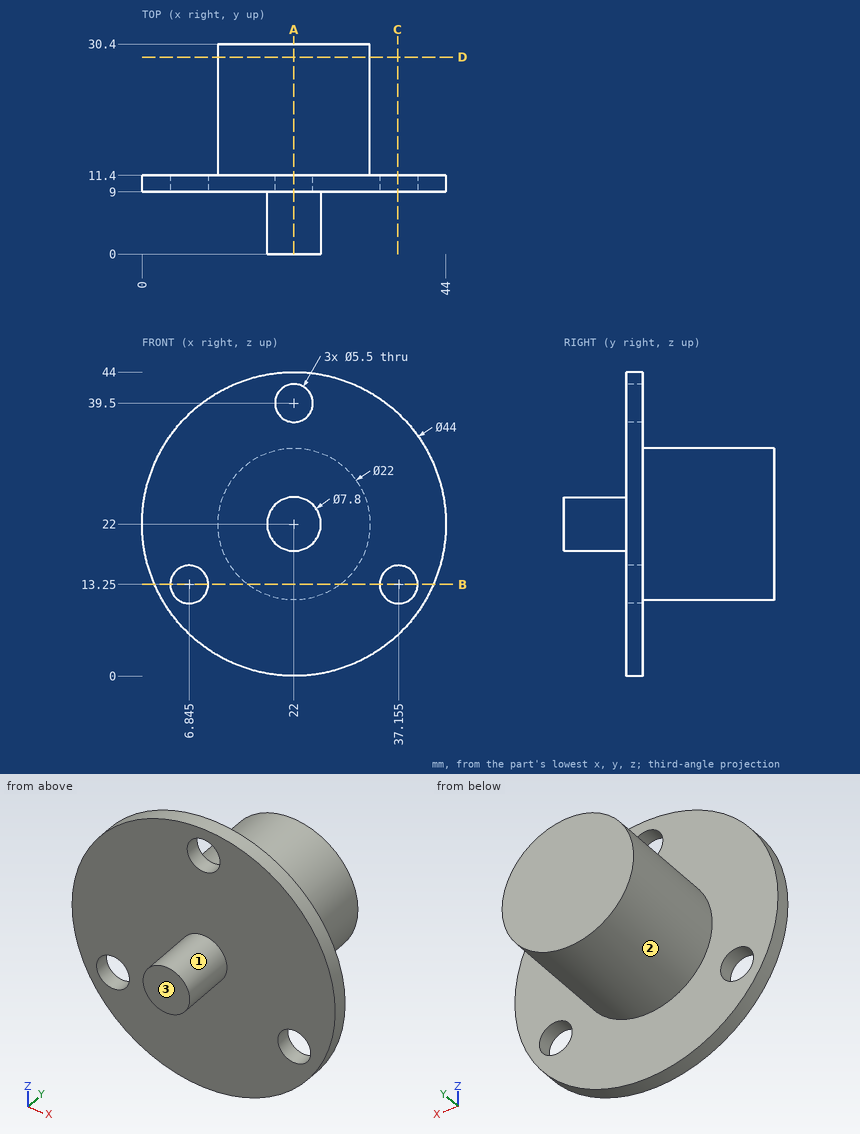
Here's the drawing with two shaded views (mm, measured from the low corner). I have some questions. A direction names the side the tool comes from. Give positions to 0.01 mm unless a question says otherwise; leave off trailing zeros. Loops run counter-clockwise (first coordinate to the right, second up) from the corner with the lowest first, then second, coordinate; pieces in that order, holes last. Notation, with made-up numbers: M -1.75,67.25 L 45.25,67.25 A28 ccw 45.25,99.25 Z; hole C 48.25,53.5 d10. An arc over 180 degrees is marked long. One line per item, written item: value.
1) Imagine slicing it at C-C on x = 37. Write out the boundary of the cut face in (y, z) (1 decimal).
Geometry check:
outline: M 9,5.9 L 11.4,5.9 L 11.4,10.5 L 9,10.5 Z; M 9,16 L 11.4,16 L 11.4,38.1 L 9,38.1 Z
2) Please list where these lines run through material, in increasing order: line 1 (Z direction, x = 22, y = 10.25); line 2 (X direction, y = 10, z = 13) (1 decimal); line 3 (Y direction, x = 15, z = 11.5).
Geometry check:
line 1: z = 0 to 36.75, 42.25 to 44
line 2: x = 1.9 to 4.1, 9.6 to 34.4, 39.9 to 42.1
line 3: y = 9 to 11.4
3) Imagine slicing it at D-D on y = 28.5. Write out the boundary of the cut face in (x, z), and give its area (3 significant figures).
Geometry check:
outline: C 22,22 d22
area: 380 mm²
4) I'm going to push flat-ended pins straight in: pin 1 (6 mm diameter, centred on x = 37, z = 36.5, fed in from +Y); pin 2 (12 mm diameter, centred on x = 6.5, y = 25, fed in from +Z) (1 decimal); pin 3 (3 mm diameter, centred on x = 32, y = 7, fed in from +Z); pin 4 (4 mm diameter, centred on y = 11, z = 27, fed in from -X) (1 decimal). Where does each tip first touch, or does it pass through?
Geometry check:
pin 1: stops at y = 11.4
pin 2: stops at z = 27.5
pin 3: passes through
pin 4: stops at x = 0.2
5) On a 3-axis mill with a long thin cutter (end or side, diameter ignored), from which of +Z, -Z, +X, -X, +Y, -Y can I reach the whole of each face in a straight line? I mean the marked faces 1, 2 and 3. Say none if no direction works.
Geometry check:
face 1: -Y
face 2: +Y
face 3: +Z, -Z, +X, -X, -Y
6) Imagine slicing it at A-A on x = 22. Write out the boundary of the cut face in (y, z).
Geometry check:
outline: M 0,18.1 L 9,18.1 L 9,0 L 11.4,0 L 11.4,11 L 30.4,11 L 30.4,33 L 11.4,33 L 11.4,36.75 L 9,36.75 L 9,25.9 L 0,25.9 Z; M 9,42.25 L 11.4,42.25 L 11.4,44 L 9,44 Z
7) Imagine slicing it at B-B on z = 13.25. Write out the boundary of the cut face in (x, y) (1 decimal).
Geometry check:
outline: M 1.8,9 L 4.1,9 L 4.1,11.4 L 1.8,11.4 Z; M 9.6,9 L 34.4,9 L 34.4,11.4 L 28.7,11.4 L 28.7,30.4 L 15.3,30.4 L 15.3,11.4 L 9.6,11.4 Z; M 39.9,9 L 42.2,9 L 42.2,11.4 L 39.9,11.4 Z
